Verification items for this drawing (mm, ordinates from the low corner). Coordinates: 2 decimals unless noted, no trailing zeros. Loops run counter-clockwise (first coordinate to the right, second up) from the corner with the lowest first, then second, coordinate; pieces in that order, holes last. Notation, with made-up numbers: (84.25, -24.5) -> (141.25, -24.5) arc R17 cw to (141.25, -11.5) -> close; hole circle Ø1 at (11.5, 79). An arc over 180 degrees is marked (long way). Write item = value, one per line.
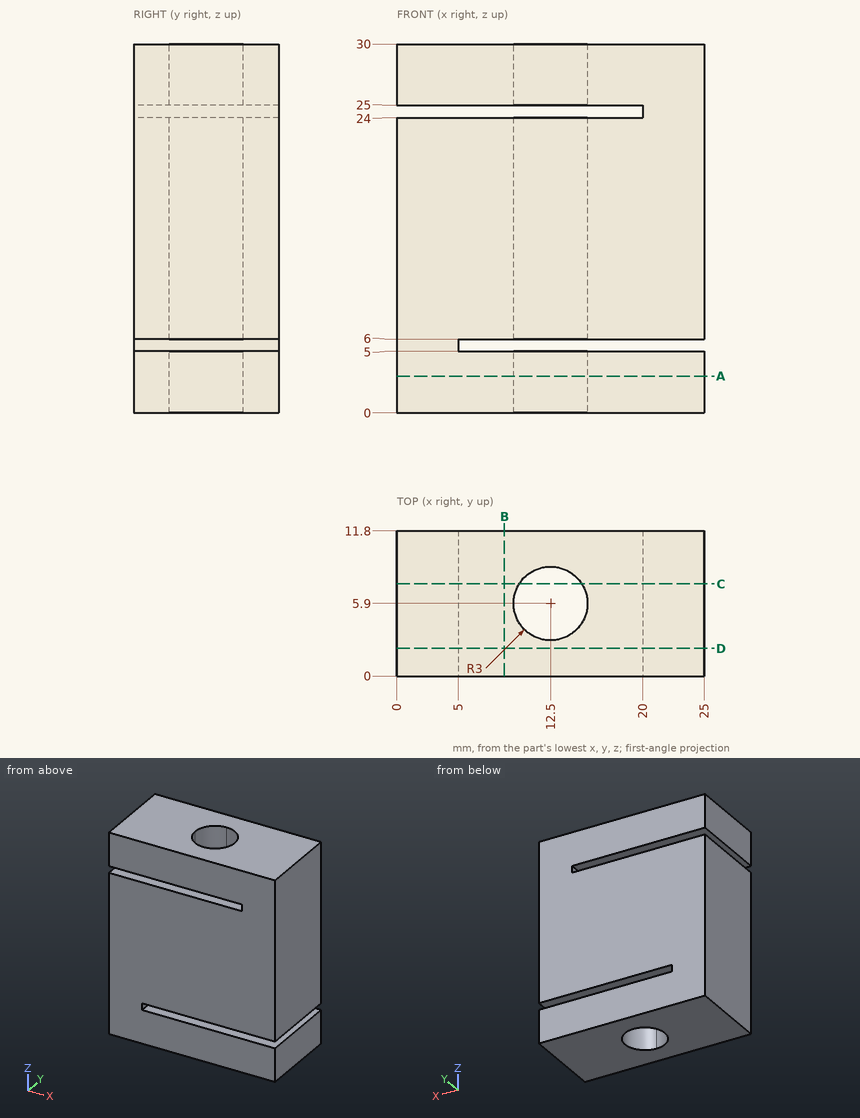
1) Sectioned sample at C-C, the plane y = 7.5. Record the cut outline in (x, z), plus the area to 3 significant figures.
Ans:
outline = (0, 0) -> (9.96, 0) -> (9.96, 5) -> (5, 5) -> (5, 6) -> (9.96, 6) -> (9.96, 24) -> (0, 24) -> close; (0, 25) -> (9.96, 25) -> (9.96, 30) -> (0, 30) -> close; (15.04, 0) -> (25, 0) -> (25, 5) -> (15.04, 5) -> close; (15.04, 6) -> (25, 6) -> (25, 30) -> (15.04, 30) -> (15.04, 25) -> (20, 25) -> (20, 24) -> (15.04, 24) -> close
area = 568 mm2
2) Sectioned sample at D-D, the plane y = 2.25. Record the cut outline in (x, z).
Ans:
outline = (0, 0) -> (25, 0) -> (25, 5) -> (5, 5) -> (5, 6) -> (25, 6) -> (25, 30) -> (0, 30) -> (0, 25) -> (20, 25) -> (20, 24) -> (0, 24) -> close
3) Depth check by flat-ended pin: pin 1 Ø0.5 at (y, z) = (3.5, 24.5) entering from -X; pin 2 Ø4 at (x, y) = (19.5, 5) entering from -Z. Enter the tip coordinate at first touch or a pass-through.
Ans:
pin_1 = 20
pin_2 = 0
4) Sectioned sample at B-B, the plane x = 8.75. Record the cut outline in (y, z), plus the area to 3 significant figures.
Ans:
outline = (0, 0) -> (11.8, 0) -> (11.8, 5) -> (0, 5) -> close; (0, 6) -> (11.8, 6) -> (11.8, 24) -> (0, 24) -> close; (0, 25) -> (11.8, 25) -> (11.8, 30) -> (0, 30) -> close
area = 330 mm2
5) Sectioned sample at A-A, the plane z = 3. Record the cut outline in (x, y), plus the area to 3 significant figures.
Ans:
outline = (0, 0) -> (25, 0) -> (25, 11.8) -> (0, 11.8) -> close; hole circle Ø6 at (12.5, 5.9)
area = 267 mm2
6) Material ranges on line 1 (Z direction, x = 14.25, y = 2); line 2 (Z direction, x = 20.5, y = 2); line 3 (X direction, y = 5.75, z = 17.75), recorded low to high.
Ans:
line_1 = 0 to 5, 6 to 24, 25 to 30
line_2 = 0 to 5, 6 to 30
line_3 = 0 to 9.5, 15.5 to 25
